```python
from build123d import *

# Parameters (mm, degrees)
SKETCH2_W                     = 49.3395
SKETCH2_H                     = 31.5341
SKETCH2_W_2                   = 44.2595
SKETCH2_H_2                   = 26.4541
BOSS_EXTRUDE1_DEPTH           = 1.905
SKETCH2_3_W                   = 49.3395
SKETCH2_3_H                   = 31.5341
SKETCH2_3_W_2                 = 44.2595
SKETCH2_3_H_2                 = 26.4541
BOSS_EXTRUDE2_DEPTH           = 9.6901
BOSS_EXTRUDE4_DEPTH           = 11.5951
CUT_EXTRUDE1_DEPTH            = 6.35
SKETCH6_R                     = 1.5
CUT_EXTRUDE2_DEPTH            = 3.429
SKETCH9_R                     = 1
BOSS_EXTRUDE6_DEPTH           = 2.794
BOSS_EXTRUDE6_DRAFT           = 2
BOSS_EXTRUDE6_PROFILE_2_DEPTH = 2.794
BOSS_EXTRUDE6_PROFILE_2_DRAFT = 2
SKETCH10_W                    = 17.4244
SKETCH10_H                    = 7.142607
CUT_EXTRUDE3_DEPTH            = 2.54
SKETCH11_W                    = 18.161
SKETCH11_H                    = 7.142607
CUT_EXTRUDE4_DEPTH            = 2.54
FILLET1_R                     = 2.54
FILLET2_R                     = 1.27
FILLET3_R                     = 2.54


with BuildPart() as part:
    # Sketch2 → Boss-Extrude1 (new body)
    # profile 1 of 2: a face of its own
    with BuildSketch(Plane(origin=(-16.248832885, 1.905, 5.92599481), x_dir=(1, 0, 0), z_dir=(0, 1, 0))):
        Rectangle(SKETCH2_W, SKETCH2_H)
        Rectangle(SKETCH2_W_2, SKETCH2_H_2, mode=Mode.SUBTRACT)
    # profile 2 of 2: a face of its own
    with BuildSketch(Plane(origin=(-16.248832885, 1.905, 5.92599481), x_dir=(1, 0, 0), z_dir=(0, 1, 0))):
        Rectangle(SKETCH2_W_2, SKETCH2_H_2)
    extrude(amount=BOSS_EXTRUDE1_DEPTH)

    # Sketch2<3> → Boss-Extrude2 (add)
    with BuildSketch(Plane(origin=(-16.248832885, 1.905, 5.92599481), x_dir=(1, 0, 0), z_dir=(0, 1, 0))):
        Rectangle(SKETCH2_3_W, SKETCH2_3_H)
        Rectangle(SKETCH2_3_W_2, SKETCH2_3_H_2, mode=Mode.SUBTRACT)
    extrude(amount=-BOSS_EXTRUDE2_DEPTH)

    # Sketch4 → Boss-Extrude4 (add)
    with BuildSketch(Plane.XZ.offset(7.7851)):
        with BuildLine():
            Line((-40.918582885, -9.84105519), (-40.918582885, -8.642431999))
            ThreePointArc((-40.918582885, -8.642431999), (-43.945507331, -12.145771785), (-39.503803797, -10.839276102))
            ThreePointArc((-39.503803797, -10.839276102), (-39.558461814, -10.328598033), (-39.719959694, -9.84105519))
            Line((-39.719959694, -9.84105519), (-40.918582885, -9.84105519))
        make_face()
        with BuildLine():
            ThreePointArc((-39.719959694, -9.84105519), (-40.210555134, -9.133027439), (-40.918582885, -8.642431999))
            Line((-40.918582885, -8.642431999), (-40.918582885, -9.84105519))
            Line((-40.918582885, -9.84105519), (-39.719959694, -9.84105519))
        make_face()
        with BuildLine():
            Line((-40.918582885, -8.642431999), (-40.918582885, -5.936055787))
            ThreePointArc((-40.918582885, -5.936055787), (-45.791911037, -14.004960596), (-36.913003797, -10.839276102))
            ThreePointArc((-36.913003797, -10.839276102), (-36.938212217, -10.337638468), (-37.013583483, -9.84105519))
            Line((-37.013583483, -9.84105519), (-39.719959694, -9.84105519))
            ThreePointArc((-39.719959694, -9.84105519), (-39.558461814, -10.328598033), (-39.503803797, -10.839276102))
            ThreePointArc((-39.503803797, -10.839276102), (-43.945507331, -12.145771785), (-40.918582885, -8.642431999))
        make_face()
        with BuildLine():
            ThreePointArc((-37.013583483, -9.84105519), (-38.378582885, -7.30105519), (-40.918582885, -5.936055787))
            Line((-40.918582885, -5.936055787), (-40.918582885, -8.642431999))
            ThreePointArc((-40.918582885, -8.642431999), (-40.210555134, -9.133027439), (-39.719959694, -9.84105519))
            Line((-39.719959694, -9.84105519), (-37.013583483, -9.84105519))
        make_face()
        with BuildLine():
            Line((8.420917115, 21.69304481), (7.222293924, 21.69304481))
            ThreePointArc((7.222293924, 21.69304481), (7.712889363, 20.985017059), (8.420917115, 20.494421619))
            Line((8.420917115, 20.494421619), (8.420917115, 21.69304481))
        make_face()
        with BuildLine():
            ThreePointArc((11.832138026, 22.691265722), (8.908459957, 25.049607705), (7.222293924, 21.69304481))
            Line((7.222293924, 21.69304481), (8.420917115, 21.69304481))
            Line((8.420917115, 21.69304481), (8.420917115, 20.494421619))
            ThreePointArc((8.420917115, 20.494421619), (10.72563371, 20.662562188), (11.832138026, 22.691265722))
        make_face()
        with BuildLine():
            ThreePointArc((8.420917115, 17.788045407), (12.584822521, 18.816158482), (14.422938026, 22.691265722))
            ThreePointArc((14.422938026, 22.691265722), (8.917500393, 27.669857302), (4.515917712, 21.69304481))
            Line((4.515917712, 21.69304481), (7.222293924, 21.69304481))
            ThreePointArc((7.222293924, 21.69304481), (8.908459957, 25.049607705), (11.832138026, 22.691265722))
            ThreePointArc((11.832138026, 22.691265722), (10.72563371, 20.662562188), (8.420917115, 20.494421619))
            Line((8.420917115, 20.494421619), (8.420917115, 17.788045407))
        make_face()
        with BuildLine():
            Line((7.222293924, 21.69304481), (4.515917712, 21.69304481))
            ThreePointArc((4.515917712, 21.69304481), (5.880917115, 19.15304481), (8.420917115, 17.788045407))
            Line((8.420917115, 17.788045407), (8.420917115, 20.494421619))
            ThreePointArc((8.420917115, 20.494421619), (7.712889363, 20.985017059), (7.222293924, 21.69304481))
        make_face()
    extrude(amount=-BOSS_EXTRUDE4_DEPTH)

    # Sketch4<3> → Cut-Extrude1 (cut)
    with BuildSketch(Plane.XZ.offset(7.7851)):
        with BuildLine():
            Line((-40.918582885, -9.84105519), (-40.918582885, -8.642431999))
            ThreePointArc((-40.918582885, -8.642431999), (-43.945507331, -12.145771785), (-39.503803797, -10.839276102))
            ThreePointArc((-39.503803797, -10.839276102), (-39.558461814, -10.328598033), (-39.719959694, -9.84105519))
            Line((-39.719959694, -9.84105519), (-40.918582885, -9.84105519))
        make_face()
        with BuildLine():
            ThreePointArc((-39.719959694, -9.84105519), (-40.210555134, -9.133027439), (-40.918582885, -8.642431999))
            Line((-40.918582885, -8.642431999), (-40.918582885, -9.84105519))
            Line((-40.918582885, -9.84105519), (-39.719959694, -9.84105519))
        make_face()
        with BuildLine():
            Line((8.420917115, 21.69304481), (7.222293924, 21.69304481))
            ThreePointArc((7.222293924, 21.69304481), (7.712889363, 20.985017059), (8.420917115, 20.494421619))
            Line((8.420917115, 20.494421619), (8.420917115, 21.69304481))
        make_face()
        with BuildLine():
            ThreePointArc((11.832138026, 22.691265722), (8.908459957, 25.049607705), (7.222293924, 21.69304481))
            Line((7.222293924, 21.69304481), (8.420917115, 21.69304481))
            Line((8.420917115, 21.69304481), (8.420917115, 20.494421619))
            ThreePointArc((8.420917115, 20.494421619), (10.72563371, 20.662562188), (11.832138026, 22.691265722))
        make_face()
    extrude(amount=-CUT_EXTRUDE1_DEPTH, mode=Mode.SUBTRACT)

    # Sketch6 → Cut-Extrude2 (cut)
    with BuildSketch(Plane.XZ.offset(1.4351)):
        with Locations(Location((9.419138026, 22.691265722, 0), (0, 0, 270))):
            Circle(SKETCH6_R)
        with Locations(Location((-41.916803797, -10.839276102, 0), (0, 0, 270))):
            Circle(SKETCH6_R)
    extrude(amount=-CUT_EXTRUDE2_DEPTH, mode=Mode.SUBTRACT)

    # Sketch7 → Cut-Revolve1 (revolve, cut)
    with BuildSketch(Plane(origin=(0, 0, -10.839276102), x_dir=(0, -1, 0), z_dir=(0, 0, -1)), mode=Mode.PRIVATE) as cut_revolve1_sk:
        Polygon((1.4351, 43.597127469), (7.7851, 44.716803797), (7.7851, 41.916803797), (1.4351, 41.916803797), align=None)
    revolve(cut_revolve1_sk.sketch.rotate(Axis((-41.916803797, -7.7851, -10.839276102), (0, 1, 0)), 270), axis=Axis((-41.916803797, -7.7851, -10.839276102), (0, 1, 0)), mode=Mode.SUBTRACT)

    # Sketch8 → Cut-Revolve2 (revolve, cut)
    with BuildSketch(Plane(origin=(9.419138026, 0, 0), x_dir=(0, -1, 0), z_dir=(-1, 0, 0)), mode=Mode.PRIVATE) as cut_revolve2_sk:
        Polygon((1.4351, 24.371589394), (7.7851, 25.491265722), (7.7851, 22.691265722), (1.4351, 22.691265722), align=None)
    revolve(cut_revolve2_sk.sketch.rotate(Axis((9.419138026, -7.7851, 22.691265722), (0, 1, 0)), 180), axis=Axis((9.419138026, -7.7851, 22.691265722), (0, 1, 0)), mode=Mode.SUBTRACT)


with BuildPart() as boss_extrude6_tool:
    # Sketch9 → Boss-Extrude6 (with draft: the straight prism first)
    with BuildSketch(Plane.XZ.offset(-1.905)):
        with Locations((-35.108582885, 15.88304481)):
            Circle(SKETCH9_R)
    extrude(amount=BOSS_EXTRUDE6_DEPTH)
    # Boss-Extrude6: the draft: its side faces are tilted about the plane it starts from
    boss_extrude6_sides = [boss_extrude6_tool.faces().sort_by_distance(p)[0] for p in [
        (-36.108582885, 0.508, 15.88304481),
    ]]
    draft(boss_extrude6_sides, Plane.XZ.offset(-1.905), BOSS_EXTRUDE6_DRAFT)


with BuildPart() as part_1:
    add(part.part)

    # Boss-Extrude6: add boss_extrude6_tool
    add(boss_extrude6_tool.part)


with BuildPart() as boss_extrude6_profile_2_tool:
    # Sketch9 → Boss-Extrude6 profile 2 (with draft: the straight prism first)
    with BuildSketch(Plane.XZ.offset(-1.905)):
        with Locations((2.610917115, -4.03105519)):
            Circle(SKETCH9_R)
    extrude(amount=BOSS_EXTRUDE6_PROFILE_2_DEPTH)
    # Boss-Extrude6 profile 2: the draft: its side faces are tilted about the plane it starts from
    boss_extrude6_profile_2_sides = [boss_extrude6_profile_2_tool.faces().sort_by_distance(p)[0] for p in [
        (1.610917115, 0.508, -4.03105519),
    ]]
    draft(boss_extrude6_profile_2_sides, Plane.XZ.offset(-1.905), BOSS_EXTRUDE6_PROFILE_2_DRAFT)


with BuildPart() as part_2:
    add(part_1.part)

    # Boss-Extrude6 profile 2: add boss_extrude6_profile_2_tool
    add(boss_extrude6_profile_2_tool.part)

    # Sketch10 → Cut-Extrude3 (cut)
    with BuildSketch(Plane(origin=(8.420917115, 0, 0), x_dir=(0, 0, -1), z_dir=(1, 0, 0))):
        with Locations((-5.92599481, -4.2137965)):
            Rectangle(SKETCH10_W, SKETCH10_H)
    extrude(amount=-CUT_EXTRUDE3_DEPTH, mode=Mode.SUBTRACT)

    # Sketch11 → Cut-Extrude4 (cut)
    with BuildSketch(Plane.ZY.offset(40.918582885)):
        with Locations((5.92599481, -4.2137965)):
            Rectangle(SKETCH11_W, SKETCH11_H)
    extrude(amount=-CUT_EXTRUDE4_DEPTH, mode=Mode.SUBTRACT)

    # Fillet1
    fillet1_edges = [part_2.edges().sort_by_distance(p)[0] for p in [
        (-40.918582885, -1.98755, 21.69304481),
        (8.420917115, -1.98755, -9.84105519),
    ]]
    fillet(fillet1_edges, radius=FILLET1_R)

    # Fillet2
    fillet2_edges = [part_2.edges().sort_by_distance(p)[0] for p in [
        (-38.378582885, -2.94005, 19.15304481),
        (5.880917115, -2.94005, 19.15304481),
        (5.880917115, -2.94005, -7.30105519),
        (-38.378582885, -2.94005, -7.30105519),
    ]]
    fillet(fillet2_edges, radius=FILLET2_R)

    # Fillet3
    fillet3_edges = [part_2.edges().sort_by_distance(p)[0] for p in [
        (-37.013583483, -1.98755, -9.84105519),
        (-40.918582885, -1.98755, -5.936055787),
        (4.515917712, -1.98755, 21.69304481),
        (8.420917115, -1.98755, 17.788045407),
    ]]
    fillet(fillet3_edges, radius=FILLET3_R)


solid = part_2.part
```
Can you work these out from the model? Positions are in its coordinate system, mm. A direction names the side the tool comes from. Round coordinates to 2 decimals unless told otherwise and drop trailing zeros. Order: outer loops, then holes, each group sorted by start corner. A loop starts at its lowest first (then second) coordinate and runs counter-clockwise, first axis right, second up. Notation, with made-up numbers: (87.5, -34.75) -> (107.5, -34.75) arc R18 cw to (107.5, -4.75) -> close; hole circle Ø9 at (-5.75, 77.5). An arc over 180 degrees is marked (long way). Return JSON: item names as keys, results as strings. Group by question number.
1. If we section it at A-A, the plane x = 0: Write out the boundary of the cut face in (y, z) (3 decimals), then the cut area to 3 significant figures.
2. If we section it at C-C, the plane z = 13: Write out the boundary of the cut face in (x, y) (1 decimal), then the cut area to 3 significant figures.
3. I need wall thicknesses on line 1 (Z direction, x = -19, y = -1); line 2 (X direction, y = 0, z = -3); line 3 (Z direction, x = -1, y = 2.5). Which ranges of each line are inside material? Lowest first, please. Write a range as [from, to].
4. Which directions (+Z, -Z, +X, -X, +Y, -Y) give clear straight access to the entire face, cutting with the end or side of a thin tool? Please do faces 1 (the face through (-40.919, 1, 11)), 2 (the face through (-37.997, -3.008, -6.939)), 3 (the face through (8.421, 1, 2)), 4 (the face through (-40, -4, 15.006)).
5. We'd pull the mould along Z, two halves only. Please class faces 5 (the face through (-44.42, -6.22, -10.51)), 6 (the face through (-18, -2, 21.693)), 7 (the face through (-17, 3.81, 6)): released by +Z, released by -Z, zero draft, split by the parting line, or undercut.
6. Will these pins go through, and if not, where does the flat tip stop? pin 1 (5 mm diameter, centred on x = -16.5, y = -4, fed in from -Z); pin 2 (1 mm diameter, centred on x = -35.5, y = -6, fed in from -Z); pin 3 (0.8 mm diameter, centred on x = 7, z = 4, fed in from -Y); pin 4 (4 mm diameter, centred on x = -41.5, z = -12, fed in from -Y).
7. If we section it at B-B, the plane y = -4: Count the separate pieces of the cut face and the enclosed holes in it, then the cut area to 3 significant figures.
Output values:
{
 "1": {"outline": "(-7.785, -9.841) -> (3.81, -9.841) -> (3.81, 21.693) -> (-7.785, 21.693) -> (-7.785, 19.153) -> (1.905, 19.153) -> (1.905, -7.301) -> (-7.785, -7.301) -> close", "area": "109 mm²"},
 "2": {"outline": "(-40.9, -0.6) -> (-38.4, -0.6) -> (-38.4, 1.9) -> (5.9, 1.9) -> (5.9, -0.6) -> (8.4, -0.6) -> (8.4, 3.8) -> (-40.9, 3.8) -> close", "area": "107 mm²"},
 "3": {"line 1": "[-9.84, -7.3], [19.15, 21.69]", "line 2": "[-40.92, -38.38], [5.88, 8.42]", "line 3": "[-9.84, 21.69]"},
 "4": {"face 1": "+Z, -X, +Y, -Y", "face 2": "-Y", "face 3": "-Z, +X, +Y, -Y", "face 4": "-X, -Y"},
 "5": {"face 5": "undercut", "face 6": "released by +Z", "face 7": "zero draft"},
 "6": {"pin 1": "z = -9.84", "pin 2": "z = -10.31", "pin 3": "y = -0.64", "pin 4": "y = -7.79"},
 "7": {"separate pieces": "2", "enclosed holes": "2", "area": "397 mm²"}
}
